from build123d import *

# Parameters (mm, degrees)
SKETCH1_W           = 45.72
SKETCH1_H           = 26.67
BOSS_EXTRUDE1_DEPTH = 17.78
FILLET1_R           = 1.27
SKETCH2_R           = 2.9845
SKETCH2_R_2         = 4.0005
BOSS_EXTRUDE2_DEPTH = 3.302


with BuildPart() as part:
    # Sketch1 → Boss-Extrude1 (new body)
    with BuildSketch(Plane.XY):
        Rectangle(SKETCH1_W, SKETCH1_H)
    extrude(amount=BOSS_EXTRUDE1_DEPTH)

    # Fillet1
    fillet1_edges = [part.edges().sort_by_distance(p)[0] for p in [
        (-22.86, 0, 17.78),
        (0, -13.335, 17.78),
        (22.86, 0, 17.78),
        (0, -13.335, 0),
        (-22.86, 0, 0),
        (0, 13.335, 0),
        (22.86, 0, 0),
        (0, 13.335, 17.78),
        (22.86, -13.335, 8.89),
        (-22.86, -13.335, 8.89),
        (-22.86, 13.335, 8.89),
        (22.86, 13.335, 8.89),
    ]]
    fillet(fillet1_edges, radius=FILLET1_R)

    # Sketch2 → Boss-Extrude2 (add)
    with BuildSketch(Plane.ZY.offset(22.86)):
        with Locations(Location((8.89, 6.5405, 0), (0, 0, 90))):
            Circle(SKETCH2_R)
        with Locations(Location((8.89, -5.8801, 0), (0, 0, 90))):
            Circle(SKETCH2_R_2)
    extrude(amount=BOSS_EXTRUDE2_DEPTH)


solid = part.part
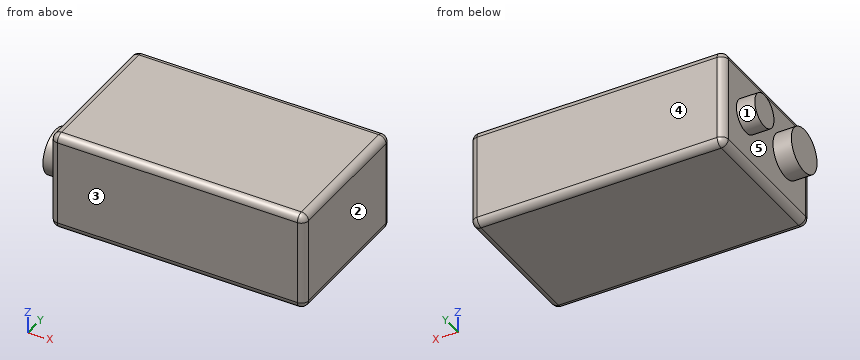
Geometry check sheet. Reference: the model listing, model coordinates, mm. Face numbers are marked on the shaded views. A direction names the side the tool comes from. Give positions to 0.01 mm unless a question says otherwise; leave off trailing zeros. Loops run counter-clockwise (first coordinate to the right, second up) from the corner with the lowest first, then second, coordinate; pieces in that order, holes last. Notation, with made-up numbers: (4, 39) -> (54, 39) arc R13 cw to (54, 46) -> close; hole circle Ø2 at (-30.75, -28.5). An arc over 180 degrees is marked (long way). Answer in a Markdown table with one row per item. Add a question column.
1) Cross-section at A-A on z = 8.89. Record the boundary of the cut face in (x, y) (3 decimals).
2) Cross-section at D-D on z = 6.75. Record the boundary of the cut face in (x, y) (3 decimals).
3) Draft check along Y on the marked faces 1, 2 and 3. Enter one of: pulls with the +Y half, pulls with the -Y half, needs draft (parallel to the pull), parting line crosses it, or undercut.
4) Cross-section at C-C on z = 15.25. Record the boundary of the cut face in (x, y) (3 decimals), and give its area (3 significant figures).
5) Cross-section at B-B on y = 7.5. Record the boundary of the cut face in (x, z), and give its area (3 significant figures).
6) Set-up check for the marked faces 4 and 5: record each of +Z, -Z, +X, -X, +Y, -Y from which the full face is reachable in a straight line by a thin tool's end or side.
7) Material ranges on probe 1 along X at (y, z) = (-10, 6.25); probe 2 along Y at (x, z) = (-22, 3.25); probe 3 along X at (y, z) = (-3, 17.25), recorded low to high. Write a range as from..to.
Outcome:
| question | item | result |
|---|---|---|
| 1 | outline | (-26.162, -9.881) -> (-22.86, -9.881) -> (-22.86, -12.065) arc R1.27 ccw to (-21.59, -13.335) -> (21.59, -13.335) arc R1.27 ccw to (22.86, -12.065) -> (22.86, 12.065) arc R1.27 ccw to (21.59, 13.335) -> (-21.59, 13.335) arc R1.27 ccw to (-22.86, 12.065) -> (-22.86, 9.525) -> (-26.162, 9.525) -> (-26.162, 3.556) -> (-22.86, 3.556) -> (-22.86, -1.88) -> (-26.162, -1.88) -> close |
| 2 | outline | (-26.162, -9.26) -> (-22.86, -9.26) -> (-22.86, -12.065) arc R1.27 ccw to (-21.59, -13.335) -> (21.59, -13.335) arc R1.27 ccw to (22.86, -12.065) -> (22.86, 12.065) arc R1.27 ccw to (21.59, 13.335) -> (-21.59, 13.335) arc R1.27 ccw to (-22.86, 12.065) -> (-22.86, 8.621) -> (-26.162, 8.621) -> (-26.162, 4.46) -> (-22.86, 4.46) -> (-22.86, -2.5) -> (-26.162, -2.5) -> close |
| 3 | face 1 | undercut |
| 3 | face 2 | needs draft |
| 3 | face 3 | pulls with the -Y half |
| 4 | outline | (-22.86, -12.065) arc R1.27 ccw to (-21.59, -13.335) -> (21.59, -13.335) arc R1.27 ccw to (22.86, -12.065) -> (22.86, 12.065) arc R1.27 ccw to (21.59, 13.335) -> (-21.59, 13.335) arc R1.27 ccw to (-22.86, 12.065) -> close |
| 4 | area | 1,220 mm^2 |
| 5 | outline | (-26.16, 6.06) -> (-22.86, 6.06) -> (-22.86, 1.27) arc R1.27 ccw to (-21.59, 0) -> (21.59, 0) arc R1.27 ccw to (22.86, 1.27) -> (22.86, 16.51) arc R1.27 ccw to (21.59, 17.78) -> (-21.59, 17.78) arc R1.27 ccw to (-22.86, 16.51) -> (-22.86, 11.72) -> (-26.16, 11.72) -> close |
| 5 | area | 830 mm^2 |
| 6 | face 4 | +Z, -Z, +X, -X, +Y |
| 6 | face 5 | -X |
| 7 | probe 1 | x = -22.86..22.86 |
| 7 | probe 2 | y = -13.27..13.27 |
| 7 | probe 3 | x = -22.62..22.62 |
